Autodesk Inventor part; units mm, degrees
ref_plane "YZ Plane" through (0, 0, 0) normal (1, 0, 0) x (0, 1, 0)
ref_plane "XZ Plane" through (0, 0, 0) normal (0, 1, 0) x (-1, 0, 0)
ref_plane "XY Plane" through (0, 0, 0) normal (0, 0, 1) x (1, 0, 0)
sketch "Sketch1" plane through (0, 0, 0) normal (0, 0, 1) x (1, 0, 0)
  circle A0 centre (0, 0) radius 3.25
extrude "Extrusion1" add sketch "Sketch1" along normal blind 1.75
sketch "Sketch2" plane through (0, 0, 1.75) normal (0, 0, 1) x (1, 0, 0)
  circle A0 centre (0, 0) radius 2.5
extrude "Extrusion2" add sketch "Sketch2" along normal blind 10
thread "Thread1"
chamfer "Chamfer1" distance 0.5 angle 45 1 edges at (-3.25, 0, 0)
properties part number "Bolt2" material "Steel, Carbon"
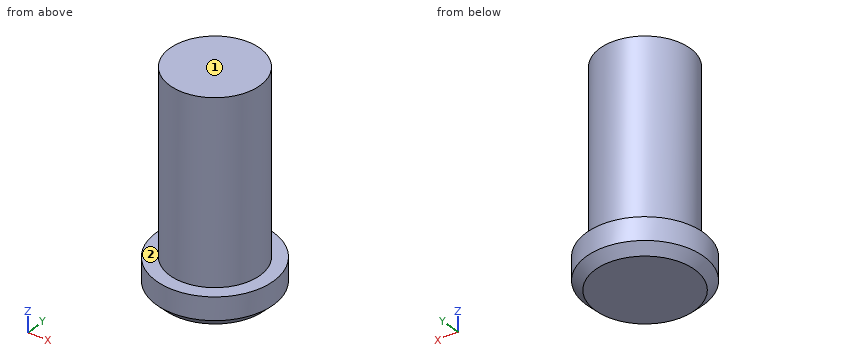
Geometry check sheet. Reference: the model listing, model coordinates, mm. Face numbers are marked on the shaded views. A direction names the side the tool comes from. Give positions to 0.01 mm unless a question says otherwise; leave off trailing zeros. Order: outer loops, then holes, each group sorted by start corner. A loop starts at its lowest first (then second) coordinate and runs counter-clockwise, first axis right, second up.
1. Scan lines: line 1 (Z direction, x = -1, y = 2.5); line 2 (Y direction, x = 0, z = 6.5); line 3 (Y direction, x = 1.75, z = 2.25). Record each from-to range of solid material in increasing order.
Completed:
line 1: z = 0 to 1.75
line 2: y = -2.5 to 2.5
line 3: y = -1.79 to 1.79
2. Depth check by flat-ended pin: pin 1 (1 mm diameter, centred on y = 2, z = 6, fed in from -X); pin 2 (2 mm diameter, centred on y = 1.5, z = 7, fed in from -X); pin 3 (2 mm diameter, centred on x = 2, z = 9, fed in from -Y). Enter the tip coordinate at first touch or a pass-through.
Completed:
pin 1: stops at x = -2
pin 2: stops at x = -2.45
pin 3: stops at y = -2.29
3. Sectioned sample at C-C (z = 7). Record the boundary of the cut face in (x, y).
Completed:
outline: circle Ø5 at (0, 0)
4. Access from +Z, -Z, +X, -X, +Y, -Y to the whole of each face (thin tool, end or side, straight path). Record for the marked faces 1 and 2.
Completed:
face 1: +Z, +X, -X, +Y, -Y
face 2: +Z
5. Sectioned sample at D-D (z = 1.5). Record the boundary of the cut face in (x, y), then the cut area to 3 significant figures.
Completed:
outline: circle Ø6.5 at (0, 0)
area: 33.2 mm2
6. Sectioned sample at A-A (y = 0). Record the boundary of the cut face in (x, z).
Completed:
outline: (-3.25, 0.5) - (-2.75, 0) - (2.75, 0) - (3.25, 0.5) - (3.25, 1.75) - (2.5, 1.75) - (2.5, 11.75) - (-2.5, 11.75) - (-2.5, 1.75) - (-3.25, 1.75) - close
